Print and shaded views of the part. All mm, measured from the part's lowest x, y and z. Give positions to 0.01 mm unless a question says otherwise; leave off trailing zeros. Loops run counter-clockwise (first coordinate to the right, second up) from the corner with the lowest first, then second, coordinate; pieces in that order, holes last. Notation, with made-up numbers: M -20.5,49.5 L 26.5,49.5 A11 ccw 26.5,57.5 Z; hole C 28,74 d11. An arc over 180 degrees is marked long. Answer in a Markdown table with one row per item.
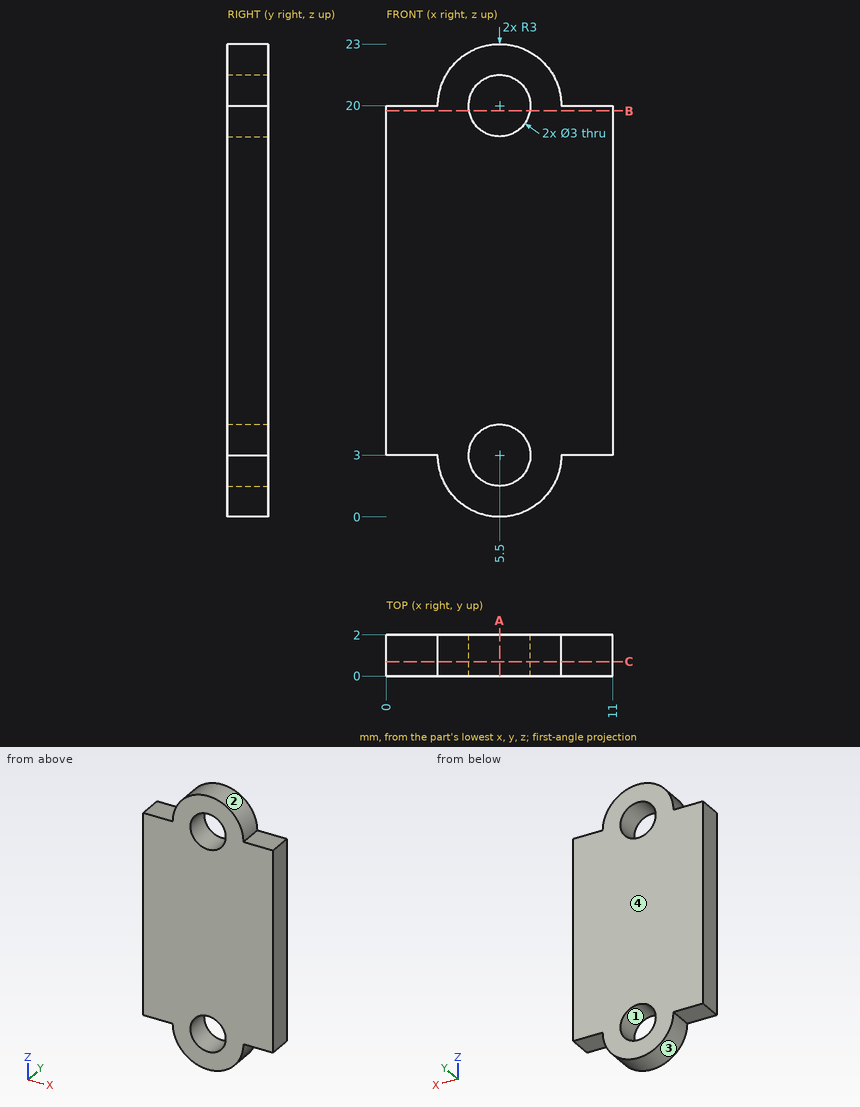
(1) Saw through at A-A, the plane x = 5.5. Give the cut face in (y, z), and give its area (3 significant figures).
Established:
| item | result |
|---|---|
| outline | M 0,0 L 2,0 L 2,1.5 L 0,1.5 Z; M 0,4.5 L 2,4.5 L 2,18.5 L 0,18.5 Z; M 0,21.5 L 2,21.5 L 2,23 L 0,23 Z |
| area | 34.0 mm2 |
(2) Saw through at B-B, the plane z = 19.75. Give the cut face in (x, y).
Established:
| item | result |
|---|---|
| outline | M 0,0 L 4.02,0 L 4.02,2 L 0,2 Z; M 6.98,0 L 11,0 L 11,2 L 6.98,2 Z |
(3) Flat gauge pins, fed straight in: P1, Ø1, axis at x = 10, y = 0.5, coming from the -Z side; P2, Ø1, axis at x = 2.5, y = 1, coming from the +Z side; P3, Ø0.6, axis at x = 9.5, y = 1.5, coming from the +Z side. Where does each tip first touch, or does it go through?
Established:
| item | result |
|---|---|
| P1 | stops at z = 3 |
| P2 | stops at z = 21.66 |
| P3 | stops at z = 20 |
(4) Mould opens along Z. For the marked faces 1, 2, 3 and 4 say: pulls with the +Z half, pulls with the -Z half, needs draft (parallel to the pull), parting line crosses it, or undercut.
Established:
| item | result |
|---|---|
| face 1 | undercut |
| face 2 | pulls with the +Z half |
| face 3 | pulls with the -Z half |
| face 4 | needs draft |
(5) Saw through at C-C, the plane y = 0.7. Give the cut face in (x, z), and give its area (3 significant figures).
Established:
| item | result |
|---|---|
| outline | M 0,3 L 2.5,3 A3 ccw 8.5,3 L 11,3 L 11,20 L 8.5,20 A3 ccw 2.5,20 L 0,20 Z; hole C 5.5,3 d3; hole C 5.5,20 d3 |
| area | 201 mm2 |
(6) Wall check: L1, parallel to Z at x = 5.5, y = 1.25; L2, parallel to Z at x = 4.5, y = 0.2; L3, parallel to Z at x = 10, y = 0.2. Give the ranges that are in metal, low to high.
Established:
| item | result |
|---|---|
| L1 | z = 0 to 1.5, 4.5 to 18.5, 21.5 to 23 |
| L2 | z = 0.17 to 1.88, 4.12 to 18.88, 21.12 to 22.83 |
| L3 | z = 3 to 20 |
